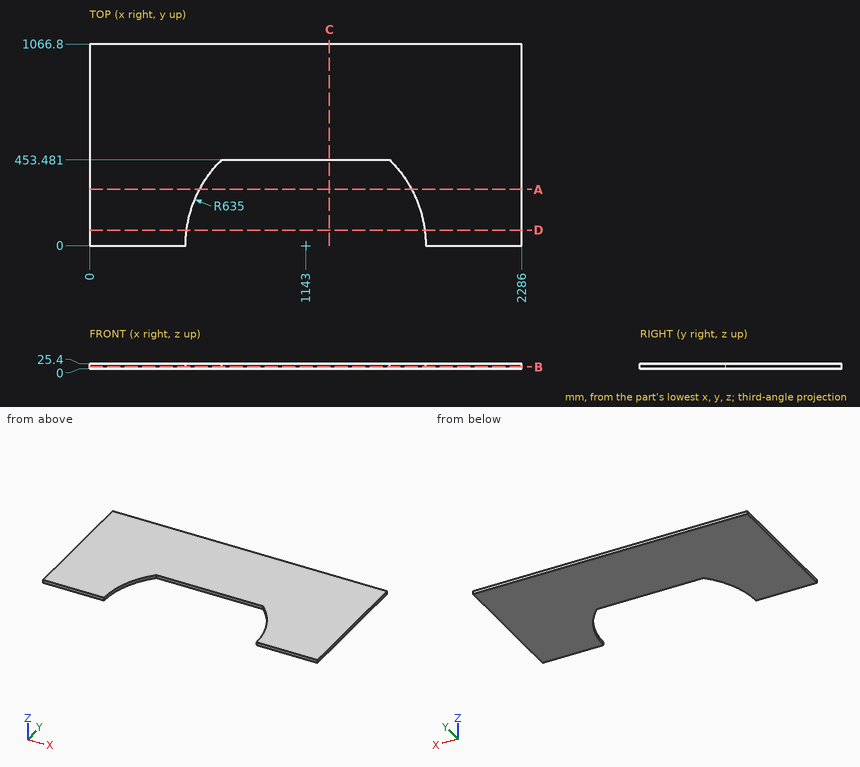
Source: three-view drawing plus pictorial views. Frame: mm from the lowest corner of the part. Round coordinates to 2 decimals unless told otherwise and drop trailing zeros. Write each loop counter-clockwise with the first axis right and the second up, starting at its lowest first coordinate (ties: lowest second). Pieces come first, ordered by that corner, then holes. Notation, with made-up numbers: (62.5, 57.5) -> (110.5, 57.5) arc R9 ccw to (110.5, 66.5) -> close; hole circle Ø3 at (-26.5, 25). An arc over 180 degrees is marked (long way). Return JSON: item names as keys, results as strings.
Q1. Section A-A on y = 297.5. Return the cut outline in (x, z), and give its area (3 significant figures).
From the geometry:
{"outline": "(0, 0) -> (582, 0) -> (582, 25.4) -> (0, 25.4) -> close; (1704, 0) -> (2286, 0) -> (2286, 25.4) -> (1704, 25.4) -> close", "area": "29,600 mm2"}
Q2. First-contact query: pin 1 Ø12.5 at (x, z) = (999, 8) entering from -Y; pin 2 Ø6 at (y, z) = (657, 5) entering from -X. Flat tips, straight axial feed; report the tip coordinate or a pass-through.
From the geometry:
{"pin 1": "y = 453.48", "pin 2": "x = 0"}
Q3. Ray query, line 1 (Y direction, x = 1546, z = 9.75); line 2 (X direction, y = 65, z = 10.75) (1 decimal); line 3 (X direction, y = 116.5, z = 12). Return the intervals inside material, ascending.
From the geometry:
{"line 1": "453.48 to 1066.8", "line 2": "0 to 511.3, 1774.7 to 2286", "line 3": "0 to 518.78, 1767.22 to 2286"}
Q4. Section D-D on y = 82. Return the cut outline in (x, z).
From the geometry:
{"outline": "(0, 0) -> (513.32, 0) -> (513.32, 25.4) -> (0, 25.4) -> close; (1772.68, 0) -> (2286, 0) -> (2286, 25.4) -> (1772.68, 25.4) -> close"}
Q5. Section C-C on x = 1268. Return the cut outline in (y, z), and give its area (3 significant figures).
From the geometry:
{"outline": "(453.48, 0) -> (1066.8, 0) -> (1066.8, 25.4) -> (453.48, 25.4) -> close", "area": "15,600 mm2"}
Q6. Section B-B on z = 9. Return the cut outline in (x, y), and give its area (3 significant figures).
From the geometry:
{"outline": "(0, 0) -> (508, 0) arc R635 cw to (698.5, 453.48) -> (1587.5, 453.48) arc R635 cw to (1778, 0) -> (2286, 0) -> (2286, 1066.8) -> (0, 1066.8) -> close", "area": "1,920,000 mm2"}
